from build123d import *

# Parameters (mm, degrees)
SKETCH2_W           = 104.14
SKETCH2_H           = 33.02
BOSS_EXTRUDE1_DEPTH = 5.334
CAVITY1_START       = 0.4826
CAVITY1_DEPTH       = 4.8514
CAVITY1_2_OUTLINE_R = 12.8016
CAVITY1_2_DEPTH     = 0.4826


# Read off the part's stored shape, not the designer's step: Cavity1
with BuildPart() as part:
    # Sketch2 → Boss-Extrude1 (new body)
    with BuildSketch(Plane.XY):
        with Locations((52.07, 16.51)):
            Rectangle(SKETCH2_W, SKETCH2_H)
    extrude(amount=BOSS_EXTRUDE1_DEPTH)

    # Cavity1 outline → Cavity1 (cut)
    with BuildSketch(Plane.XY.offset(CAVITY1_START)):
        with BuildLine():
            Line((73.183671361, 33.02), (17.000497532, 33.02))
            Line((17.000497532, 33.02), (54.31426706, 8.129320565))
            ThreePointArc((54.31426706, 8.129320565), (76.777861535, 10.697572054), (73.183671361, 33.02))
        make_face()
    extrude(amount=CAVITY1_DEPTH, mode=Mode.SUBTRACT)

    # Cavity1 2 outline → Cavity1 2 (cut)
    with BuildSketch(Plane.XY):
        with Locations((64.319453414, 20.142181246)):
            Circle(CAVITY1_2_OUTLINE_R)
    extrude(amount=CAVITY1_2_DEPTH, mode=Mode.SUBTRACT)


solid = part.part
Geometry check sheet. Reference: the model listing, model coordinates, mm. A direction names the side the tool comes from. Round coordinates to 2 decimals unless told otherwise and drop trailing zeros. Loops run counter-clockwise (first coordinate to the right, second up) from the corner with the lowest first, then second, coordinate; pieces in that order, holes last.
Item 1: Mould release check, pull along Y, two halves, no side actions. Record for faces 1 (the cylindrical face through (76.56, 10.42, 2.87)), 2 (the flat face through (35.396, 20.749, 2.874)), 3 (the flat face through (104.14, 16, 3)), 4 (the flat face through (51, 0, 3)): pulls with the +Y half, pulls with the -Y half, needs draft (parallel to the pull), parting line crosses it, or undercut.
Item 2: Cross-section at D-D on z = 3.1. Record the boundary of the cut face in (x, y), then the cut area to 3 significant figures.
Item 3: Access from +Z, -Z, +X, -X, +Y, -Y to the whole of each face (thin tool, end or side, straight path). Record for faces 5 (the cylindrical face through (76.53, 23.99, 0.24)), 6 (the flat face through (48, 22, 0.483)).
Item 4: Gauge pin test, flat ends, axial feed: pin 1 (1.5 mm diameter, centred on x = 91, z = 4, fed in from -Y); pin 2 (1.5 mm diameter, centred on x = 18.5, z = 2, fed in from +Y). Record the tip position at first contact, or that the pin passes through.
Item 5: Cross-section at C-C on y = 22. Record the boundary of the cut face in (x, z).
Item 6: Thickness scan on line 1 (X direction, y = 26.5, z = 0.45); line 2 (X direction, y = 27, z = 4.55); line 3 (Y direction, x = 76, z = 1.7). Record the ranges inside material, lowest first.
Item 7: Cross-section at B-B on x = 68.5. Record the boundary of the cut face in (y, z), then the cut area to 3 significant figures.
Item 8: Cross-section at A-A on y = 31. Record the boundary of the cut face in (x, z).
Answer sheet:
1. face 1: undercut
1. face 2: pulls with the +Y half
1. face 3: needs draft
1. face 4: pulls with the -Y half
2. outline: (0, 0) - (104.14, 0) - (104.14, 33.02) - (73.18, 33.02) arc R15.63 cw (long way) to (54.31, 8.13) - (17, 33.02) - (0, 33.02) - close
2. area: 2,330 mm2
3. face 5: +Z, -Z
3. face 6: +Z
4. pin 1: stops at y = 0
4. pin 2: stops at y = 32.52
5. outline: (0, 0) - (51.65, 0) - (51.65, 0.48) - (33.52, 0.48) - (33.52, 5.33) - (0, 5.33) - close; (76.99, 0) - (104.14, 0) - (104.14, 5.33) - (79.84, 5.33) - (79.84, 0.48) - (76.99, 0.48) - close
6. line 1: x = 0 to 53.21, 75.43 to 104.14
6. line 2: x = 0 to 26.03, 78.37 to 104.14
6. line 3: y = 0 to 9.75, 30.53 to 33.02
7. outline: (0, 0) - (8.04, 0) - (8.04, 0.48) - (5.08, 0.48) - (5.08, 5.33) - (0, 5.33) - close; (32.24, 0) - (33.02, 0) - (33.02, 0.48) - (32.24, 0.48) - close
7. area: 28.9 mm2
8. outline: (0, 0) - (57.54, 0) - (57.54, 0.48) - (20.03, 0.48) - (20.03, 5.33) - (0, 5.33) - close; (71.1, 0) - (104.14, 0) - (104.14, 5.33) - (75.57, 5.33) - (75.57, 0.48) - (71.1, 0.48) - close
